from build123d import *

# Parameters (mm, degrees)
SCHIZZO1_R                   = 15
SCHIZZO1_R_2                 = 2.89
ESTRUSIONE_ESTRUSIONE1_DEPTH = 4
TAGLIO_ESTRUSIONE1_DEPTH     = 22.587033145


with BuildPart() as part:
    # Schizzo1 → Estrusione-Estrusione1 (new body)
    with BuildSketch(Plane.XY):
        Circle(SCHIZZO1_R)
        Circle(SCHIZZO1_R_2, mode=Mode.SUBTRACT)
    extrude(amount=ESTRUSIONE_ESTRUSIONE1_DEPTH)

    # Schizzo2 → Taglio-Estrusione1 (cut, through all)
    with BuildSketch(Plane.XY.offset(4)):
        with BuildLine():
            Line((-4.829629131, -1.294095226), (-11.108147002, -2.976419019))
            ThreePointArc((-11.108147002, -2.976419019), (-11.5, 0), (-11.108147002, 2.976419019))
            Line((-11.108147002, 2.976419019), (-4.829629131, 1.294095226))
            ThreePointArc((-4.829629131, 1.294095226), (-5, 0), (-4.829629131, -1.294095226))
        make_face()
        with BuildLine():
            Line((11.108147002, -2.976419019), (4.829629131, -1.294095226))
            ThreePointArc((4.829629131, -1.294095226), (5, 0), (4.829629131, 1.294095226))
            Line((4.829629131, 1.294095226), (11.108147002, 2.976419019))
            ThreePointArc((11.108147002, 2.976419019), (11.5, 0), (11.108147002, -2.976419019))
        make_face()
        with BuildLine():
            Line((-2.976419019, 11.108147002), (-1.294095226, 4.829629131))
            ThreePointArc((-1.294095226, 4.829629131), (0, 5), (1.294095226, 4.829629131))
            Line((1.294095226, 4.829629131), (2.976419019, 11.108147002))
            ThreePointArc((2.976419019, 11.108147002), (0, 11.5), (-2.976419019, 11.108147002))
        make_face()
        with BuildLine():
            Line((-2.976419019, -11.108147002), (-1.294095226, -4.829629131))
            ThreePointArc((-1.294095226, -4.829629131), (0, -5), (1.294095226, -4.829629131))
            Line((1.294095226, -4.829629131), (2.976419019, -11.108147002))
            ThreePointArc((2.976419019, -11.108147002), (0, -11.5), (-2.976419019, -11.108147002))
        make_face()
    extrude(amount=-TAGLIO_ESTRUSIONE1_DEPTH, mode=Mode.SUBTRACT)


solid = part.part
Input: part model. Units: mm. Frame: model coordinates. A direction names the side the tool comes from. Give positions to 0.01 mm unless a question says otherwise; leave off trailing zeros. Loops run counter-clockwise (first coordinate to the right, second up) from the corner with the lowest first, then second, coordinate; pieces in that order, holes last. Notation, with made-up numbers: (-14, 76.5) -> (26, 76.5) arc R25 ccw to (26, 98.5) -> close; hole circle Ø3 at (-25, -22.5). An arc over 180 degrees is marked (long way). Answer as a JSON object with one key per item and string values. Group by question number.
Item 1: Cut plane C-C, the plane z = 3.6. Return the cut outline in (x, y), and give its area (3 significant figures).
Item 2: Cut plane A-A, the plane x = 0. Return the cut outline in (y, z).
Item 3: Pull-direction query (Y, two-part tool) for faces 3 (the cylindrical face through (-14.985, 0.66, 1.972)), 4 (the cylindrical face through (-5, 0, 2)), 5 (the flat face through (-8.013, 2.147, 2.028)), 6 (the flat face through (3.1, 0.2, 4)); classes: released by +Y, released by -Y, zero draft, split by the parting line, or undercut.
Item 4: Line query: probe 1 along Y at (x, z) = (-1, 3.05); probe 2 along X at (y, z) = (-1.25, 2.1); probe 3 along Y at (x, z) = (9.5, 3.05). Output: solid intervals per line, ascending.
Item 5: Pin query (flat end, axial travel): P1, Ø1.5, axis at x = 11.5, z = 0.5, coming from the -Y side; P2, Ø2, axis at y = 10, z = 1.5, coming from the +X side; P3, Ø3.5, axis at x = 0, y = 0, coming from the -Z side. Return the tip coordinate at first contact, or that it passes through.
Item 6: Cut plane D-D, the plane y = 8.25. Return the cut outline in (x, z).
Item 7: Reachability of faces 1 (the cylindrical face through (0, -5, 2)), 2 (the flat face through (3.1, 0.2, 0)) from +Z, -Z, +X, -X, +Y, -Y: full face, straight path, thin tool, end or side. Return the list, or none.
Checks:
{
 "1": {"outline": "circle Ø30 at (0, 0); hole (-11.11, -2.98) -> (-4.83, -1.29) arc R5 cw to (-4.83, 1.29) -> (-11.11, 2.98) arc R11.5 ccw to start; hole (-2.98, -11.11) arc R11.5 ccw to (2.98, -11.11) -> (1.29, -4.83) arc R5 cw to (-1.29, -4.83) -> close; hole (-2.98, 11.11) -> (-1.29, 4.83) arc R5 cw to (1.29, 4.83) -> (2.98, 11.11) arc R11.5 ccw to start; hole circle Ø5.78 at (0, 0); hole (4.83, -1.29) -> (11.11, -2.98) arc R11.5 ccw to (11.11, 2.98) -> (4.83, 1.29) arc R5 cw to start", "area": "568 mm²"},
 "2": {"outline": "(-15, 0) -> (-11.5, 0) -> (-11.5, 4) -> (-15, 4) -> close; (-5, 0) -> (-2.89, 0) -> (-2.89, 4) -> (-5, 4) -> close; (2.89, 0) -> (5, 0) -> (5, 4) -> (2.89, 4) -> close; (11.5, 0) -> (15, 0) -> (15, 4) -> (11.5, 4) -> close"},
 "3": {"face 3": "split by the parting line", "face 4": "undercut", "face 5": "undercut", "face 6": "zero draft"},
 "4": {"probe 1": "y = -14.97 to -11.46, -4.9 to -2.71, 2.71 to 4.9, 11.46 to 14.97", "probe 2": "x = -14.95 to -11.43, -4.84 to -2.61, 2.61 to 4.84, 11.43 to 14.95", "probe 3": "y = -11.61 to -2.55, 2.55 to 11.61"},
 "5": {"P1": "stops at y = -10.46", "P2": "stops at x = 12", "P3": "passes through"},
 "6": {"outline": "(-12.53, 0) -> (-2.21, 0) -> (-2.21, 4) -> (-12.53, 4) -> close; (2.21, 0) -> (12.53, 0) -> (12.53, 4) -> (2.21, 4) -> close"},
 "7": {"face 1": "+Z, -Z", "face 2": "-Z, +X, -X, +Y, -Y"}
}
